from build123d import *

# Parameters (mm, degrees)
F0_W     = 57.5
F0_H     = 60.5
F0_R     = 1.5
F0_R_2   = 2.5
F0_R_3   = 6.1
F0_W_2   = 3
F0_H_2   = 7
F0_W_3   = 37.5
F0_H_3   = 33
F0_R_4   = 2
F1_DEPTH = 3.5
F3_W     = 37.5
F3_H     = 33
F3_W_2   = 33.5
F3_H_2   = 29
F4_DEPTH = 1
F2_W     = 15.5
F2_H     = 3.75
F5_DEPTH = 2.5


with BuildPart() as f1:
    # F0 (on Top) → F1 (new body)
    with BuildSketch(Plane.XY):
        with Locations((94.6610440163, 0)):
            Rectangle(F0_W, F0_H)
        with Locations((68.9110440163, -27.25)):
            Circle(F0_R, mode=Mode.SUBTRACT)
        with Locations((89.6610440163, -23)):
            Circle(F0_R, mode=Mode.SUBTRACT)
        with Locations((80.5132240057, -18.15)):
            Circle(F0_R_2, mode=Mode.SUBTRACT)
        with Locations((109.3110440163, -18.15)):
            Circle(F0_R_3, mode=Mode.SUBTRACT)
        with Locations((117.1610440163, -2)):
            Rectangle(F0_W_2, F0_H_2, mode=Mode.SUBTRACT)
        with Locations((94.6610440163, 10)):
            Rectangle(F0_W_3, F0_H_3, mode=Mode.SUBTRACT)
        with Locations((117.1610440163, 8.5)):
            Circle(F0_R_4, mode=Mode.SUBTRACT)
        with Locations((120.4110440163, 27.25)):
            Circle(F0_R, mode=Mode.SUBTRACT)
    extrude(amount=F1_DEPTH)

    # F3 (on face) → F4 (join)
    with BuildSketch(Plane(origin=(0, 0, 0), x_dir=(1, 0, 0), z_dir=(0, 0, -1))):
        with Locations((94.6610440163, -10)):
            Rectangle(F3_W, F3_H)
        with Locations((94.6610440163, -10)):
            Rectangle(F3_W_2, F3_H_2, mode=Mode.SUBTRACT)
    extrude(amount=-F4_DEPTH)

    # F2 (on face) → F5 (cut)
    with BuildSketch(Plane.XY.offset(3.5)):
        with Locations((94.6610440163, 28.375)):
            Rectangle(F2_W, F2_H)
    extrude(amount=-F5_DEPTH, mode=Mode.SUBTRACT)


solid = f1.part
The model under review builds one solid part; all positions refer to its coordinate system, in mm. A direction names the side the tool comes from. Give positions to 0.01 mm unless a question says otherwise; leave off trailing zeros. Loops run counter-clockwise (first coordinate to the right, second up) from the corner with the lowest first, then second, coordinate; pieces in that order, holes last. Notation, with made-up numbers: (75, -15.5) -> (87, -15.5) arc R15 ccw to (87, -4.5) -> close; hole circle Ø1 at (11, 1.25). An arc over 180 degrees is marked (long way). Answer as a JSON object with one key per item and string values. Group by question number.
Q1. Take a section at D-D (y = -2). Write out the cut boundary in (x, z).
Q2. Take a section at A-A (y = -18.15). Write out the cut boundary in (x, z), plus the area to 3 significant figures.
Q3. Insertion check: pin 1 (4.5 mm diameter, centred on x = 80.51, y = -18.15, fed in from -Z); pin 2 (0.8 mm diameter, centred on x = 87.5, z = 2, fed in from +Y). Each pin has a flat end and moves straight along its axis. Give the tip position at first contact, or say it passes through.
Q4. Take a section at B-B (z = 1.8). Write out the cut boundary in (x, y).
Q5. Draft analysis for pull direction X (two halves, no side actions). For faces 6 (the flat face through (94.3, 30.25, 0.6)), 7 (the flat face through (123.411, 0, 2)), 8 (the cylindrical face through (91.09, -22.55, 1.73)), state which applies: pulls with the +X half, pulls with the -X half, needs draft (parallel to the pull), parting line crosses it, or undercut.
Q6. Wall thickness on line 1 along Y through (x, z) = (86, 2.3); line 2 along X through (y, z) = (13, 2.65); line 3 along Y through (x, z) = (95, 0.65): over which ranges is each line inside the solid? List them lowest first.
Q7. Take a section at C-C (y = 23.5). Write out the cut boundary in (x, z), plus the area to 3 significant figures.
Q8. Tool access review of faces 1 (the flat face through (94, -6.5, 2)), 2 (the flat face through (94, -30.25, 2)), 3 (the flat face through (102.411, 28, 2)), 4 (the flat face through (94, -7, 0)), 5 (the flat face through (118.661, -2, 2)): name each direction out of +Z, -Z, +X, -X, +Y, -Y from which nothing blocks a thin tool from reaching the whole face with its end or side.
Answer below:
{
 "1": {"outline": "(65.91, 0) -> (77.91, 0) -> (77.91, 1) -> (75.91, 1) -> (75.91, 3.5) -> (65.91, 3.5) -> close; (111.41, 0) -> (115.66, 0) -> (115.66, 3.5) -> (113.41, 3.5) -> (113.41, 1) -> (111.41, 1) -> close; (118.66, 0) -> (123.41, 0) -> (123.41, 3.5) -> (118.66, 3.5) -> close"},
 "2": {"outline": "(65.91, 0) -> (78.01, 0) -> (78.01, 3.5) -> (65.91, 3.5) -> close; (83.01, 0) -> (103.21, 0) -> (103.21, 3.5) -> (83.01, 3.5) -> close; (115.41, 0) -> (123.41, 0) -> (123.41, 3.5) -> (115.41, 3.5) -> close", "area": "141 mm2"},
 "3": {"pin 1": "passes through", "pin 2": "stops at y = -6.5"},
 "4": {"outline": "(65.91, -30.25) -> (123.41, -30.25) -> (123.41, 30.25) -> (102.41, 30.25) -> (102.41, 26.5) -> (113.41, 26.5) -> (113.41, -6.5) -> (75.91, -6.5) -> (75.91, 26.5) -> (86.91, 26.5) -> (86.91, 30.25) -> (65.91, 30.25) -> close; hole circle Ø3 at (68.91, -27.25); hole circle Ø5 at (80.51, -18.15); hole circle Ø3 at (89.66, -23); hole circle Ø12.2 at (109.31, -18.15); hole circle Ø4 at (117.16, 8.5); hole (115.66, -5.5) -> (118.66, -5.5) -> (118.66, 1.5) -> (115.66, 1.5) -> close; hole circle Ø3 at (120.41, 27.25)"},
 "5": {"face 6": "needs draft", "face 7": "pulls with the +X half", "face 8": "undercut"},
 "6": {"line 1": "y = -30.25 to -6.5, 26.5 to 30.25", "line 2": "x = 65.91 to 75.91, 113.41 to 123.41", "line 3": "y = -30.25 to -4.5, 24.5 to 30.25"},
 "7": {"outline": "(65.91, 0) -> (77.91, 0) -> (77.91, 1) -> (75.91, 1) -> (75.91, 3.5) -> (65.91, 3.5) -> close; (111.41, 0) -> (123.41, 0) -> (123.41, 3.5) -> (113.41, 3.5) -> (113.41, 1) -> (111.41, 1) -> close", "area": "74.0 mm2"},
 "8": {"face 1": "+Z", "face 2": "+Z, -Z, +X, -X, -Y", "face 3": "+Z, +Y", "face 4": "-Z, +X, -X, +Y, -Y", "face 5": "+Z, -Z"}
}
